Input: dimensioned drawing with shaded views. Units: mm. Origin: part minimum x, y, z. A direction names the side the tool comes from. Give positions to 0.01 mm unless a question says otherwise; leave off trailing zeros. Write each loop counter-clockwise with the first axis right and the second up, starting at its lowest first coordinate (ties: lowest second). Pieces come first, ordered by that corner, then holes.
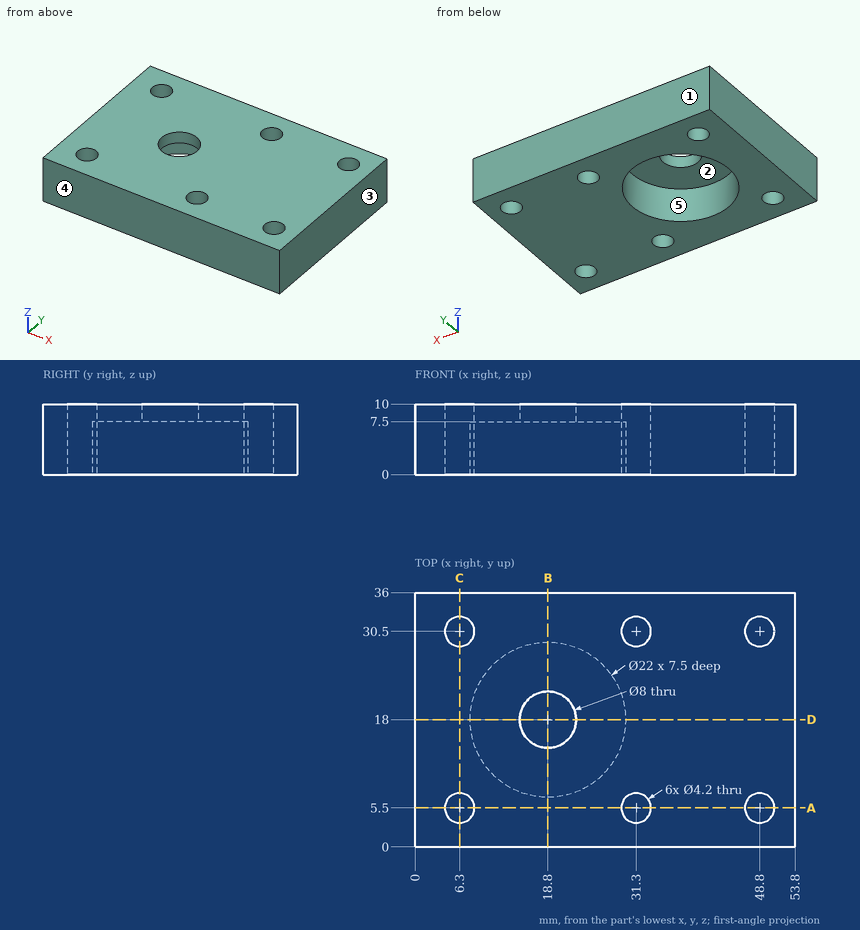
Item 1: Section C-C (x = 6.3). Return loops of the section in (y, z).
Item 2: Section D-D (y = 18). Return loops of the section in (x, z), and give its area (3 significant figures).
Item 3: Section A-A (y = 5.5). Return loops of the section in (x, z), and give its area (3 significant figures).
Item 4: Mould query, pull axis Y, two halves, no side actions, for the marked faces 1, 2 and 3. Classes: +Y half, -Y half, draft (parallel to the pull), parting line (faces both ways), or undercut.
Item 5: Ray query, line 1 (Y direction, x = 48.8, z = 6.25); line 2 (Y direction, x = 18.8, z = 2); line 3 (X direction, y = 31, z = 2). Return the intervals inside material, ascending.
Item 6: Section B-B (x = 18.8). Return loops of the section in (y, z).
Item 7: Pin query (flat end, axial travel): pin 1 (17.5 mm diameter, centred on x = 17.5, y = 18, fed in from -Z); pin 2 (4 mm diameter, centred on x = 6.3, y = 5.5, fed in from -Z). Return the tip coordinate at first contact, or that it passes through.
Item 8: Set-up query: the marked faces 4 and 5. Return all of +Z, -Z, +X, -X, +Y, -Y with unobstructed straight access to the full face (end or side cutting, diameter ignored); none if empty.
Solved:
1. outline: (0, 0) - (3.4, 0) - (3.4, 10) - (0, 10) - close; (7.6, 0) - (28.4, 0) - (28.4, 10) - (7.6, 10) - close; (32.6, 0) - (36, 0) - (36, 10) - (32.6, 10) - close
2. outline: (0, 0) - (7.8, 0) - (7.8, 7.5) - (14.8, 7.5) - (14.8, 10) - (0, 10) - close; (22.8, 7.5) - (29.8, 7.5) - (29.8, 0) - (53.8, 0) - (53.8, 10) - (22.8, 10) - close
2. area: 353 mm2
3. outline: (0, 0) - (4.2, 0) - (4.2, 10) - (0, 10) - close; (8.4, 0) - (29.2, 0) - (29.2, 10) - (8.4, 10) - close; (33.4, 0) - (46.7, 0) - (46.7, 10) - (33.4, 10) - close; (50.9, 0) - (53.8, 0) - (53.8, 10) - (50.9, 10) - close
3. area: 412 mm2
4. face 1: +Y half
4. face 2: undercut
4. face 3: draft
5. line 1: y = 0 to 3.4, 7.6 to 28.4, 32.6 to 36
5. line 2: y = 0 to 7, 29 to 36
5. line 3: x = 0 to 4.26, 8.34 to 29.26, 33.34 to 46.76, 50.84 to 53.8
6. outline: (0, 0) - (7, 0) - (7, 7.5) - (14, 7.5) - (14, 10) - (0, 10) - close; (22, 7.5) - (29, 7.5) - (29, 0) - (36, 0) - (36, 10) - (22, 10) - close
7. pin 1: stops at z = 7.5
7. pin 2: passes through
8. face 4: +Z, -Z, +X, -X, -Y
8. face 5: -Z
